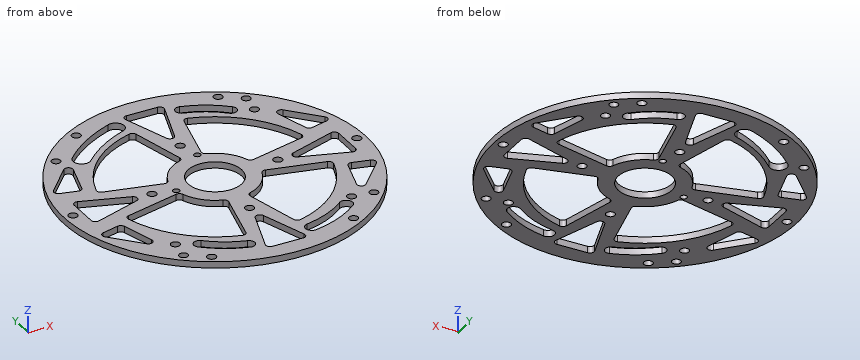
```python
from build123d import *

# Parameters (mm, degrees)
SKETCH_1_R          = 70.64
SKETCH_1_R_2        = 2.1
SKETCH_1_R_3        = 1.55
EXTRUDE_1_DEPTH     = 3
SKETCH_2_R          = 12.5
CUT_EXTRUDE_1_DEPTH = 100.945080919
SKETCH_5_R          = 2.05
CUT_EXTRUDE_2_DEPTH = 100.945080919
CUT_EXTRUDE_3_DEPTH = 100.945080919
FILLET_1_R          = 2
CUT_EXTRUDE_4_DEPTH = 100.945080919


with BuildPart() as part:
    # 草图1 → 凸台-拉伸1 (new body)
    with BuildSketch(Plane.XY):
        Circle(SKETCH_1_R)
        with Locations((41.308177097, 41.308177097)):
            Circle(SKETCH_1_R_2, mode=Mode.SUBTRACT)
        with Locations((33.25, 57.590689352)):
            Circle(SKETCH_1_R_2, mode=Mode.SUBTRACT)
        with Locations((66.5, 0)):
            Circle(SKETCH_1_R_2, mode=Mode.SUBTRACT)
        with Locations((33.25, -57.590689352)):
            Circle(SKETCH_1_R_2, mode=Mode.SUBTRACT)
        with Locations((-33.25, -57.590689352)):
            Circle(SKETCH_1_R_2, mode=Mode.SUBTRACT)
        with Locations((-66.5, 0)):
            Circle(SKETCH_1_R_2, mode=Mode.SUBTRACT)
        with Locations((-33.25, 57.590689352)):
            Circle(SKETCH_1_R_2, mode=Mode.SUBTRACT)
        with Locations((41.308177097, -41.308177097)):
            Circle(SKETCH_1_R_2, mode=Mode.SUBTRACT)
        with Locations((-41.308177097, -41.308177097)):
            Circle(SKETCH_1_R_2, mode=Mode.SUBTRACT)
        with Locations((0, -29.5)):
            Circle(SKETCH_1_R_2, mode=Mode.SUBTRACT)
        with Locations((-29.5, 0)):
            Circle(SKETCH_1_R_2, mode=Mode.SUBTRACT)
        with Locations((0, 29.5)):
            Circle(SKETCH_1_R_2, mode=Mode.SUBTRACT)
        with Locations((29.5, 0)):
            Circle(SKETCH_1_R_2, mode=Mode.SUBTRACT)
        with Locations((2.474873734, 19.445436483)):
            Circle(SKETCH_1_R_3, mode=Mode.SUBTRACT)
        with Locations((-19.445436483, -2.474873734)):
            Circle(SKETCH_1_R_3, mode=Mode.SUBTRACT)
    extrude(amount=EXTRUDE_1_DEPTH)

    # 草图2 → 切除-拉伸1 (cut, through all)
    with BuildSketch(Plane.XY.offset(3)):
        Circle(SKETCH_2_R)
    extrude(amount=-CUT_EXTRUDE_1_DEPTH, mode=Mode.SUBTRACT)

    # 草图5 → 切除-拉伸2 (cut, through all)
    with BuildSketch(Plane.XY.offset(3)):
        with Locations((-50.941955467, 42.745376044)):
            Circle(SKETCH_5_R)
        with Locations((42.745376044, 50.941955467)):
            Circle(SKETCH_5_R)
        with Locations((50.941955467, -42.745376044)):
            Circle(SKETCH_5_R)
        with Locations((-42.745376044, -50.941955467)):
            Circle(SKETCH_5_R)
    extrude(amount=-CUT_EXTRUDE_2_DEPTH, mode=Mode.SUBTRACT)

    # 草图6 → 切除-拉伸3 (cut, through all)
    with BuildSketch(Plane.XY.offset(3)):
        with BuildLine():
            Line((-4.576065072, 19.060682791), (-11.672268193, 48.61849602))
            ThreePointArc((-11.672268193, 48.61849602), (-35.355339059, 35.355339059), (-48.61849602, 11.672268193))
            Line((-48.61849602, 11.672268193), (-19.060682791, 4.576065072))
            ThreePointArc((-19.060682791, 4.576065072), (-13.860916276, 13.860916276), (-4.576065072, 19.060682791))
        make_face()
        with BuildLine():
            Line((19.060682791, 4.576065072), (48.61849602, 11.672268193))
            ThreePointArc((48.61849602, 11.672268193), (35.355339059, 35.355339059), (11.672268193, 48.61849602))
            Line((11.672268193, 48.61849602), (4.576065072, 19.060682791))
            ThreePointArc((4.576065072, 19.060682791), (13.860916276, 13.860916276), (19.060682791, 4.576065072))
        make_face()
        with BuildLine():
            Line((4.576065072, -19.060682791), (11.672268193, -48.61849602))
            ThreePointArc((11.672268193, -48.61849602), (35.355339059, -35.355339059), (48.61849602, -11.672268193))
            Line((48.61849602, -11.672268193), (19.060682791, -4.576065072))
            ThreePointArc((19.060682791, -4.576065072), (13.860916276, -13.860916276), (4.576065072, -19.060682791))
        make_face()
        with BuildLine():
            Line((-19.060682791, -4.576065072), (-48.61849602, -11.672268193))
            ThreePointArc((-48.61849602, -11.672268193), (-35.355339059, -35.355339059), (-11.672268193, -48.61849602))
            Line((-11.672268193, -48.61849602), (-4.576065072, -19.060682791))
            ThreePointArc((-4.576065072, -19.060682791), (-13.860916276, -13.860916276), (-19.060682791, -4.576065072))
        make_face()
        Polygon((-10, 62), (10, 62), (0, 32), align=None)
        Polygon((32, 0), (62, 10), (62, -10), align=None)
        Polygon((0, -32), (10, -62), (-10, -62), align=None)
        Polygon((-32, 0), (-62, -10), (-62, 10), align=None)
        Polygon((52.962057119, -16.209483435), (65.903980805, -19.41411476), (45.635039833, -41.568110983), align=None)
        Polygon((65.903980805, 19.41411476), (45.635039833, 41.568110983), (52.962057119, 16.209483435), align=None)
        Polygon((-52.962057119, 16.209483435), (-65.903980805, 19.41411476), (-45.635039833, 41.568110983), align=None)
        Polygon((-65.903980805, -19.41411476), (-45.635039833, -41.568110983), (-52.962057119, -16.209483435), align=None)
    extrude(amount=-CUT_EXTRUDE_3_DEPTH, mode=Mode.SUBTRACT)

    # 圆角1
    fillet_1_edges = [part.edges().sort_by_distance(p)[0] for p in [
        (45.635039833, -41.568110983, 1.5),
        (52.962057119, -16.209483435, 1.5),
        (65.903980805, -19.41411476, 1.5),
        (65.903980805, 19.41411476, 1.5),
        (52.962057119, 16.209483435, 1.5),
        (45.635039833, 41.568110983, 1.5),
        (62, 10, 1.5),
        (62, -10, 1.5),
        (32, 0, 1.5),
        (10, -62, 1.5),
        (-10, -62, 1.5),
        (0, -32, 1.5),
        (-19.060682791, -4.576065072, 1.5),
        (-4.576065072, -19.060682791, 1.5),
        (-11.672268193, -48.61849602, 1.5),
        (-48.61849602, -11.672268193, 1.5),
        (4.576065072, -19.060682791, 1.5),
        (19.060682791, -4.576065072, 1.5),
        (48.61849602, -11.672268193, 1.5),
        (11.672268193, -48.61849602, 1.5),
        (19.060682791, 4.576065072, 1.5),
        (4.576065072, 19.060682791, 1.5),
        (11.672268193, 48.61849602, 1.5),
        (48.61849602, 11.672268193, 1.5),
        (-4.576065072, 19.060682791, 1.5),
        (-19.060682791, 4.576065072, 1.5),
        (-48.61849602, 11.672268193, 1.5),
        (-11.672268193, 48.61849602, 1.5),
        (-62, -10, 1.5),
        (-62, 10, 1.5),
        (-32, 0, 1.5),
        (-45.635039833, 41.568110983, 1.5),
        (-52.962057119, 16.209483435, 1.5),
        (-65.903980805, 19.41411476, 1.5),
        (-65.903980805, -19.41411476, 1.5),
        (-52.962057119, -16.209483435, 1.5),
        (-45.635039833, -41.568110983, 1.5),
        (0, 32, 1.5),
        (-10, 62, 1.5),
        (10, 62, 1.5),
    ]]
    fillet(fillet_1_edges, radius=FILLET_1_R)

    # 草图7 → 切除-拉伸4 (cut, through all)
    with BuildSketch(Plane.XY.offset(3)):
        with BuildLine():
            ThreePointArc((-17.422756273, 59.11797816), (-31.534910164, 52.05319727), (-43.737820568, 42.045550485))
            ThreePointArc((-43.737820568, 42.045550485), (-43.665129254, 36.389163301), (-38.008742071, 36.461854615))
            ThreePointArc((-38.008742071, 36.461854615), (-27.180807487, 45.341879226), (-14.658755443, 51.610628467))
            ThreePointArc((-14.658755443, 51.610628467), (-12.287081012, 56.746303729), (-17.422756273, 59.11797816))
        make_face()
        with BuildLine():
            ThreePointArc((34.460401115, 47.535925761), (25.648718973, 54.040105851), (15.460227519, 58.058157956))
            ThreePointArc((15.460227519, 58.058157956), (12.091312412, 56.039363778), (14.11010659, 52.670448672))
            ThreePointArc((14.11010659, 52.670448672), (22.957846175, 49.181151084), (30.609957309, 43.532886872))
            ThreePointArc((30.609957309, 43.532886872), (34.536698657, 43.609184414), (34.460401115, 47.535925761))
        make_face()
        with BuildLine():
            ThreePointArc((-34.220407145, -47.753045621), (-25.429192431, -54.105658673), (-15.397477434, -58.229472799))
            ThreePointArc((-15.397477434, -58.229472799), (-12.011807829, -56.321247176), (-13.920033452, -52.935577571))
            ThreePointArc((-13.920033452, -52.935577571), (-22.756252751, -49.303205044), (-30.499804191, -43.707643162))
            ThreePointArc((-30.499804191, -43.707643162), (-34.382806898, -43.870042915), (-34.220407145, -47.753045621))
        make_face()
        with BuildLine():
            ThreePointArc((15.323186317, -58.543330734), (27.442964192, -54.741609142), (38.256000225, -48.076749461))
            ThreePointArc((38.256000225, -48.076749461), (38.718203216, -43.846142313), (34.487596067, -43.383939322))
            ThreePointArc((34.487596067, -43.383939322), (24.944035587, -49.266328992), (14.247147792, -52.621719636))
            ThreePointArc((14.247147792, -52.621719636), (11.824361505, -56.120544448), (15.323186317, -58.543330734))
        make_face()
    extrude(amount=-CUT_EXTRUDE_4_DEPTH, mode=Mode.SUBTRACT)


solid = part.part
```
Could you check a few things on this model? Use its own coordinates, in mm. Give positions to 0.01 mm unless a question says otherwise; leave off trailing zeros. Write each loop counter-clockwise with the first axis right and the second up, starting at its lowest first coordinate (ties: lowest second). Pieces come first, ordered by that corner, then holes. Notation, with made-up numbers: (23, -17.5) -> (70, -17.5) arc R16 ccw to (70, 1.5) -> close; hole circle Ø9 at (77.5, -12). An arc over 180 degrees is marked (long way). Write each question's results on one line, items separated by ' | '.
1. I want a section at A-A, the plane x = 66.5. Write out the boundary of the cut face in (y, z), then the cut area to 3 significant figures.
Check sheet entries:
outline: (-23.83, 0) -> (-2.1, 0) -> (-2.1, 3) -> (-23.83, 3) -> close; (2.1, 0) -> (23.83, 0) -> (23.83, 3) -> (2.1, 3) -> close | area: 130 mm²
2. I want a section at D-D, the plane z = 0.95. Count the separate pieces of the cut face and the enclosed holes in it, then the cut area to 3 significant figures.
Check sheet entries:
separate pieces: 1 | enclosed holes: 36 | area: 7,760 mm²
3. I need wall thicknesses on L1, parallel to Y at x = -22, z = 0.65; L2, parallel to X at y = -50, z = 2.8; L3, parallel to X at y = 15.5, z = 2.5. Which ranges of each line are inside material? Lowest first, please.
Check sheet entries:
L1: y = -67.13 to -55.83, -49.71 to -44.9, -5.28 to 5.28, 44.9 to 48.36, 57.25 to 67.13 | L2: x = -49.9 to -44.57, -40.92 to -31.59, -21.45 to -6, 6 to 23.25, 35.7 to 49.9 | L3: x = -68.92 to -47.54, -12 to 12, 47.54 to 68.92
4. Will these pins go through, and if not, where does the flat tip stop? pin 1 Ø3.5 at (x, y) = (2.47, 19.45) entering from +Z; pin 2 Ø1.5 at (x, z) = (3.5, 2) entering from -Y; pin 3 Ø0.9 at (y, z) = (1, 1) entering from +X.
Check sheet entries:
pin 1: stops at z = 3 | pin 2: stops at y = -70.59 | pin 3: stops at x = 70.64
5. I want a section at B-B, the plane y = 29.5. Write out the boundary of the cut face in (x, z), then the cut area to 3 significant figures.
Check sheet entries:
outline: (-64.19, 0) -> (-56.68, 0) -> (-56.68, 3) -> (-64.19, 3) -> close; (-49.12, 0) -> (-40.37, 0) -> (-40.37, 3) -> (-49.12, 3) -> close; (-7.08, 0) -> (-2.1, 0) -> (-2.1, 3) -> (-7.08, 3) -> close; (2.1, 0) -> (7.08, 0) -> (7.08, 3) -> (2.1, 3) -> close; (40.37, 0) -> (49.12, 0) -> (49.12, 3) -> (40.37, 3) -> close; (56.68, 0) -> (64.19, 0) -> (64.19, 3) -> (56.68, 3) -> close | area: 127 mm²
6. I want a section at C-C, the plane x = 25.5. Write out the boundary of the cut face in (y, z), then the cut area to 3 significant figures.
Check sheet entries:
outline: (-65.88, 0) -> (-55.58, 0) -> (-55.58, 3) -> (-65.88, 3) -> close; (-49.01, 0) -> (-43.01, 0) -> (-43.01, 3) -> (-49.01, 3) -> close; (-6.12, 0) -> (6.12, 0) -> (6.12, 3) -> (-6.12, 3) -> close; (43.01, 0) -> (47.64, 0) -> (47.64, 3) -> (43.01, 3) -> close; (54.12, 0) -> (65.88, 0) -> (65.88, 3) -> (54.12, 3) -> close | area: 135 mm²
